from build123d import *

# Parameters (mm, degrees)
BOSS_EXTRUDE1_DEPTH = 6.35


with BuildPart() as part:
    # Sketch1 → Revolve1 (revolve)
    with BuildSketch(Plane.XY, mode=Mode.PRIVATE) as revolve1_sk:
        with BuildLine():
            Line((0, 0), (13.5, 0))
            Line((13.5, 0), (13.5, 3.175))
            Line((13.5, 3.175), (10.08, 3.175))
            ThreePointArc((10.08, 3.175), (5.589871939, 5.034871939), (3.73, 9.525))
            Line((3.73, 9.525), (3.73, 11.1125))
            Line((3.73, 11.1125), (2.38125, 11.1125))
            Line((2.38125, 11.1125), (2.38125, 23.8125))
            Line((2.38125, 23.8125), (0, 23.8125))
            Line((0, 23.8125), (0, 0))
        make_face()
    revolve(revolve1_sk.sketch.rotate(Axis((0, 23.8125, 0), (0, -1, 0)), 180), axis=Axis((0, 23.8125, 0), (0, -1, 0)))

    # Sketch2 → Boss-Extrude1 (add)
    with BuildSketch(Plane.XZ):
        Polygon((7.18570145, 0), (3.592850725, 6.223), (-3.592850725, 6.223), (-7.18570145, 0), (-3.592850725, -6.223), (3.592850725, -6.223), align=None)
    extrude(amount=BOSS_EXTRUDE1_DEPTH)


solid = part.part
Can you work these out from the model? Positions are in its coordinate system, mm. A direction names the side the tool comes from. Give positions to 0.01 mm unless a question says otherwise; leave off trailing zeros. Order: outer loops, then holes, each group sorted by start corner. A loop starts at its lowest first (then second) coordinate and runs counter-clockwise, first axis right, second up. Notation, with made-up numbers: M 16,12 L 21,12 A27 ccw 21,36 Z; hole C 41,82.5 d8. An arc over 180 degrees is marked long. One line per item, written item: value.
Item 1: If we section it at D-D on y = 13.5: Write out the boundary of the cut face in (x, z), and give its area (3 significant figures).
Verdict:
outline: C 0,0 d4.76
area: 17.8 mm2
Item 2: For faces 1 (the face through (0, -3, 6.223)), 2 (the face through (-5.414, -3.131, -3.068)), 3 (the face through (-5.36, -3.13, 3.16)), 4 (the face through (0.516, 17.551, 2.325)), which set-ups out of +Z, -Z, +X, -X, +Y, -Y let a thin tool reach every point of the face, with its end or its side?
Verdict:
face 1: +Z, +X, -X, -Y
face 2: -Z, -X, -Y
face 3: +Z, -X, -Y
face 4: +Y
Item 3: If we section it at C-C on z = 10.75: Write out the boundary of the cut face in (x, y) (3 decimals), and give its area (3 significant figures).
Verdict:
outline: M -8.166,0 L 8.166,0 L 8.166,3.175 L -8.166,3.175 Z
area: 51.9 mm2
Item 4: Please list where these lines run through material, in increasing order: line 1 (X direction, y = -3, z = 6); line 2 (Y direction, x = -5.25, z = -9.75) (3 decimals); line 3 (Y direction, x = -1.75, z = 2).
Verdict:
line 1: -3.72 to 3.72
line 2: 0 to 3.175
line 3: -6.35 to 11.11
Item 5: For pin 1 (10 mm diameter, centred on x = 0, y = 6.5, fed in from +Z); pin 2 (1 mm diameter, centred on x = 1, y = 18.5, fed in from +Z); pin 3 (8 mm diameter, centred on y = 8.5, z = -6, fed in from +X); pin 4 (3 mm diameter, centred on x = 3, y = 8.5, fed in from -Z), each with a flat end and sliding along its axis, tell me the tip position at first contact or that it passes through.
Verdict:
pin 1: z = 13.5
pin 2: z = 2.33
pin 3: x = 3.94
pin 4: z = -3.6
Item 6: If we section it at A-A on y = -3.5: Write out the boundary of the cut face in (x, z), and give its area (3 significant figures).
Verdict:
outline: M -7.19,0 L -3.59,-6.22 L 3.59,-6.22 L 7.19,0 L 3.59,6.22 L -3.59,6.22 Z
area: 134 mm2
